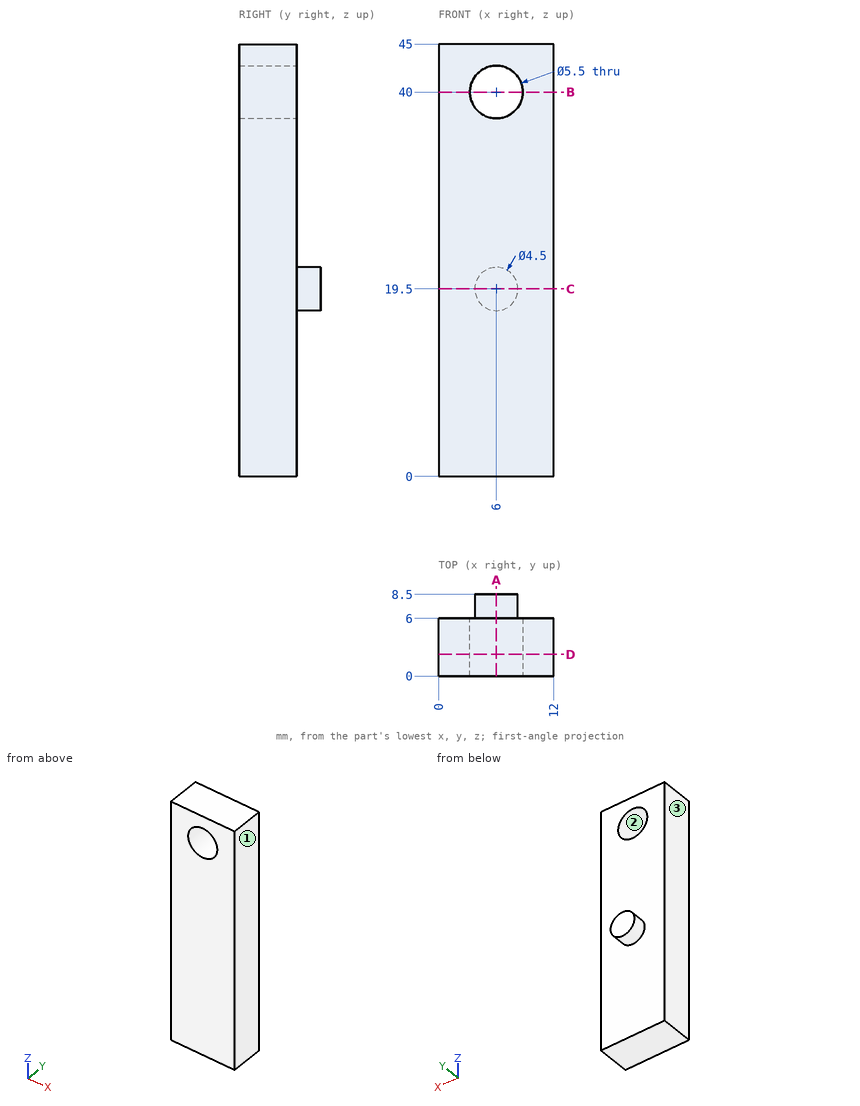
Check sheet for the drawn part. Datum: minimum x, y, z corner. Units: mm. Coordinates: 2 decimals unless noted, no trailing zeros. Loops run counter-clockwise (first coordinate to the right, second up) from the corner with the lowest first, then second, coordinate; pieces in that order, holes last. Notation, with made-up numbers: (-12, 36.25) - (-6, 36.25) arc R19 ccw to (-6, 56.25) - close; hole circle Ø6 at (75, -21.75). An arc over 180 degrees is marked (long way). Put each result on its own line as item: value.
Item 1: Scan lines: line 1 along X through (y, z) = (3.9, 40); line 2 along Z through (x, y) = (6, 1.7); line 3 along Y through (x, z) = (4, 25). Record each from-to range of solid material in increasing order.
Conclusion:
line 1: x = 0 to 3.25, 8.75 to 12
line 2: z = 0 to 37.25, 42.75 to 45
line 3: y = 0 to 6
Item 2: Section check B-B (z = 40). Enter the section's corners in (x, y), then the cut area to 3 significant figures.
Conclusion:
outline: (0, 0) - (3.25, 0) - (3.25, 6) - (0, 6) - close; (8.75, 0) - (12, 0) - (12, 6) - (8.75, 6) - close
area: 39.0 mm2
Item 3: Section check D-D (y = 2.25). Enter the section's corners in (x, z), then the cut area to 3 significant figures.
Conclusion:
outline: (0, 0) - (12, 0) - (12, 45) - (0, 45) - close; hole circle Ø5.5 at (6, 40)
area: 516 mm2
Item 4: Gauge pin test, flat end, axial feed: pin 1 Ø5 at (x, z) = (2, 38.5) entering from +Y. Record the tip position at first contact, or that the pin passes through.
Conclusion:
pin 1: stops at y = 6
Item 5: Draft check along X on the marked faces 1, 2 and 3. Enter one of: pulls with the +X half, pulls with the -X half, needs draft (parallel to the pull), parting line crosses it, or undercut.
Conclusion:
face 1: pulls with the +X half
face 2: undercut
face 3: pulls with the -X half
Item 6: Section check A-A (x = 6). Enter the section's corners in (y, z), then the cut area to 3 significant figures.
Conclusion:
outline: (0, 0) - (6, 0) - (6, 17.25) - (8.5, 17.25) - (8.5, 21.75) - (6, 21.75) - (6, 37.25) - (0, 37.25) - close; (0, 42.75) - (6, 42.75) - (6, 45) - (0, 45) - close
area: 248 mm2
Item 7: Section check C-C (z = 19.5). Enter the section's corners in (x, y).
Conclusion:
outline: (0, 0) - (12, 0) - (12, 6) - (8.25, 6) - (8.25, 8.5) - (3.75, 8.5) - (3.75, 6) - (0, 6) - close
